Verification items for the finished model (mm, model axes). Coordinates: 2 decimals unless noted, no trailing zeros. Order: outer loops, then holes, each group sorted by start corner. A loop starts at its lowest first (then second) coordinate and runs counter-clockwise, first axis right, second up. Notation, with made-up numbers: (18, 56) -> (47, 56) arc R14 cw to (47, 80) -> close; hole circle Ø2 at (86.25, 7.5). An arc over 180 degrees is marked (long way). Answer as CSV lines item,"result".
```python
from build123d import *

# Parameters (mm, degrees)
REVOLVE_1_ANGLE = 180
SKETCH_2_R      = 0.375
EXTRUDE_1_DEPTH = 10
REVOLVE_2_ANGLE = 180


with BuildPart() as part:
    # 草图1 → 旋转1 (revolve)
    with BuildSketch(Plane.XY):
        with BuildLine():
            Line((-0.5, 0), (0.5, 0))
            ThreePointArc((0.5, 0), (0, -0.5), (-0.5, 0))
        make_face()
    revolve(axis=Axis((-0.5, 0, 0), (1, 0, 0)), revolution_arc=REVOLVE_1_ANGLE)

    # 草图2 → 凸台-拉伸1 (add)
    with BuildSketch(Plane.XY):
        with Locations(Location((0, 0, 0), (0, 0, 90))):
            Circle(SKETCH_2_R)
    extrude(amount=EXTRUDE_1_DEPTH)

    # 草图3 → 旋转2 (revolve)
    with BuildSketch(Plane.XY.offset(10)):
        with BuildLine():
            Line((0, 0.5), (0, -0.5))
            ThreePointArc((0, -0.5), (-0.5, 0), (0, 0.5))
        make_face()
    revolve(axis=Axis((0, 0.5, 10), (0, 1, 0)), revolution_arc=REVOLVE_2_ANGLE)


solid = part.part
```
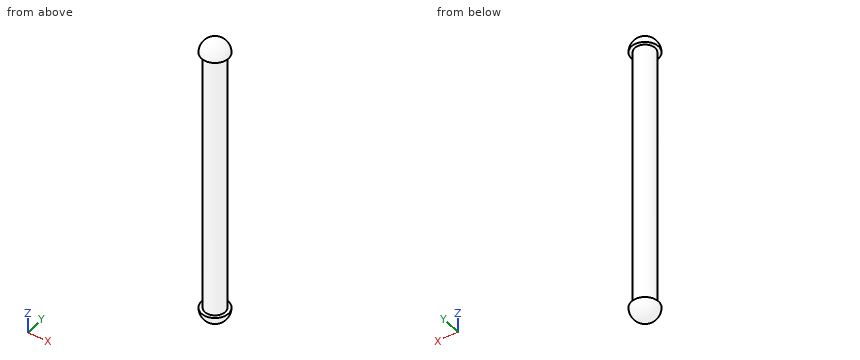
Item 1: Thickness scan on line 1 (X direction, y = 0, z = 8) (3 decimals); line 2 (Z direction, x = -0.1, y = 0.05); line 3 (X direction, y = -0.25, z = 3). Record the ranges inside material, lowest first.
Answer list:
line 1,"-0.375 to 0.375"
line 2,"-0.49 to 10.49"
line 3,"-0.28 to 0.28"
Item 2: Section check C-C, the plane z = 8.75. Record the boundary of the cut face in (x, y) (3 decimals).
Answer list:
outline,"circle Ø0.75 at (0, 0)"
Item 3: Section check A-A, the plane y = 0. Record the boundary of the cut face in (x, z) (3 decimals).
Answer list:
outline,"(-0.5, 0) arc R0.5 ccw to (0.5, 0) -> (0.375, 0) -> (0.375, 10) -> (0.5, 10) arc R0.5 ccw to (-0.5, 10) -> (-0.375, 10) -> (-0.375, 0) -> close"
